Check sheet for the modelled part. Datum: model origin and axes. Units: mm. A direction names the side the tool comes from. Give positions to 0.01 mm unless a question says otherwise; leave off trailing zeros. Order: outer loops, then holes, each group sorted by start corner. A loop starts at its lowest first (then second) coordinate and runs counter-clockwise, first axis right, second up. Notation, with made-up numbers: M 56,50 L 82,50 A14 ccw 82,72 Z; hole C -17.75,-10.5 d8. An arc over 180 degrees is marked long. Return JSON: item names as keys, results as strings. Group by question number.
Autodesk Inventor part; units mm, degrees
ref_plane "YZ Plane" through (0, 0, 0) normal (1, 0, 0) x (0, 1, 0)
ref_plane "XZ Plane" through (0, 0, 0) normal (0, 1, 0) x (-1, 0, 0)
ref_plane "XY Plane" through (0, 0, 0) normal (0, 0, 1) x (1, 0, 0)
sketch "Sketch1" plane through (0, 0, 0) normal (0, 0, 1) x (1, 0, 0)
  line L0 (0, 25.4) -> (0, -25.4)
  line L1 (0, -25.4) -> (19.05, -25.4)
  line L2 (0, 25.4) -> (19.05, 25.4)
  line L3 (19.05, 25.4) -> (19.05, 22.225)
  line L4 (19.05, 22.225) -> (3.048, 22.225)
  line L5 (3.048, 22.225) -> (3.048, -22.225)
  line L6 (3.048, -22.225) -> (19.05, -22.225)
  line L7 (19.05, -22.225) -> (19.05, -25.4)
  point P0 (0, 0)
  point P1 (0, 0)
  dimension "d0" = 50.8
  dimension "d1" = 19.05
  dimension "d2" = 3.175
  dimension "d3" = 16.002
extrude "Extrusion1" add sketch "Sketch1" along normal mid plane 660.4
fillet "Fillet1" radius 1.5875 4 edges at (3.048, 22.225, 0) (3.048, -22.225, 0) (19.05, -22.225, 0) (19.05, 22.225, 0)
sketch "Sketch2" plane through (3.048, -20.6375, -330.2) normal (1, 0, 0) x (0, 0, -1)
  point P0 (-330.2, 20.6375)
  point P1 (-177.8, 20.6375)
  point P2 (-482.6, 20.6375)
  dimension "d7" = 304.8
  dimension "d8" = 152.4
hole "Hole1" at (3.048, 0, -152.4) at (3.048, 0, 152.4) direction (-1, 0, 0) diameter 7 end through all
sketch "Sketch3" plane through (3.048, -20.6375, -330.2) normal (1, 0, 0) x (0, 0, -1)
  line L0 (-650.875, 33.3375) -> (-9.525, 33.3375)
  line L1 (-9.525, 33.3375) -> (-9.525, 7.9375)
  line L2 (-9.525, 7.9375) -> (-650.875, 7.9375)
  line L3 (-650.875, 7.9375) -> (-650.875, 33.3375)
  line L4 (-650.875, 33.3375) -> (-9.525, 7.9375) construction
  line L5 (-9.525, 33.3375) -> (-650.875, 7.9375) construction
  line L6 (0, 41.275) -> (0, 0)
  line L7 (-660.4, 0) -> (-660.4, 41.275)
  line L8 (0, -4.7625) -> (-660.4, -4.7625)
  line L9 (0, 46.0375) -> (-660.4, 46.0375)
  point P0 (-330.2, 20.6375)
  point P1 (-330.2, 7.9375)
  point P2 (-330.2, 33.3375)
  dimension "d34" = 9.525
  dimension "d35" = 9.525
  dimension "d36" = 12.7
  dimension "d37" = 12.7
hole "Hole2" at (3.048, -12.7, 320.675) at (3.048, 12.7, 320.675) at (3.048, -12.7, 0) at (3.048, 12.7, 0) at (3.048, -12.7, -320.675) at (3.048, 12.7, -320.675) direction (-1, 0, 0) diameter 5.1054 depth 25.4 tip angle 118
sketch "Sketch5" plane through (3.048, -20.6375, -330.2) normal (1, 0, 0) x (0, 0, -1)
  circle A0 centre (-482.6, 20.6375) radius 3.5
  circle A1 centre (-177.8, 20.6375) radius 3.5
  point P0 (-330.2, 20.6375)
  point P1 (-466.6, 20.6375)
  point P2 (-498.6, 20.6375)
  point P3 (-193.8, 20.6375)
  point P4 (-161.8, 20.6375)
  dimension "d23" = 32
  dimension "d24" = 16
  dimension "d25" = 32
  dimension "d26" = 16
hole "Hole3" at (3.048, 0, 168.4) at (3.048, 0, 136.4) at (3.048, 0, -136.4) at (3.048, 0, -168.4) direction (-1, 0, 0) diameter 4.4958 end through all
equation "\"d4\" = Length"
equation "\"Length\" = 660.4"
properties part number "NASA-20-FR-OP-01" material "Aluminum 6061"
1) Depth check by flat-ended pin: P1, Ø5, axis at y = 10, z = -188.5, coming from the +X side; P2, Ø5.5, axis at y = 0, z = -152.4, coming from the +X side. Enter the tip coordinate at first touch or a pass-through.
2) Release check for a two-part mould opening along Y. For faces 1 (the face through (3.048, 0, -5)), 2 (the face through (2, 2, 330.2)), 3 (the face through (9, 25.4, -5)), 4 (the face through (9, -25.4, -5)) record: released by +Y, released by -Y, zero draft, split by the parting line, or undercut.
3) Material ranges on line 1 along Y through (x, z) = (2.25, 0); line 2 along Y through (x, z) = (15.75, -242.5) (3 decimals); line 3 along Y through (x, z) = (2, 152.4), recorded low to high.
4) Tool access check on faces 5 (the face through (0, 0, -5)), 6 (the face through (11, 22.225, -5)). Record the directions out of +Z, -Z, +X, -X, +Y, -Y that give a thin tool (end or side, any length) a straight path to the whole face; none if there is none.
5) Sectioned sample at A-A on x = 8.25. Record the boundary of the cut face in (y, z) (3 decimals).
Reply:
{
 "1": {"P1": "x = 3.05", "P2": "through"},
 "2": {"face 1": "undercut", "face 2": "zero draft", "face 3": "released by +Y", "face 4": "released by -Y"},
 "3": {"line 1": "-25.4 to -15.25, -10.15 to 10.15, 15.25 to 25.4", "line 2": "-25.4 to -22.225, 22.225 to 25.4", "line 3": "-25.4 to -3.5, 3.5 to 25.4"},
 "4": {"face 5": "+Z, -Z, -X, +Y, -Y", "face 6": "+Z, -Z, +X"},
 "5": {"outline": "M -25.4,-330.2 L -22.225,-330.2 L -22.225,330.2 L -25.4,330.2 Z; M 22.225,-330.2 L 25.4,-330.2 L 25.4,330.2 L 22.225,330.2 Z"}
}
